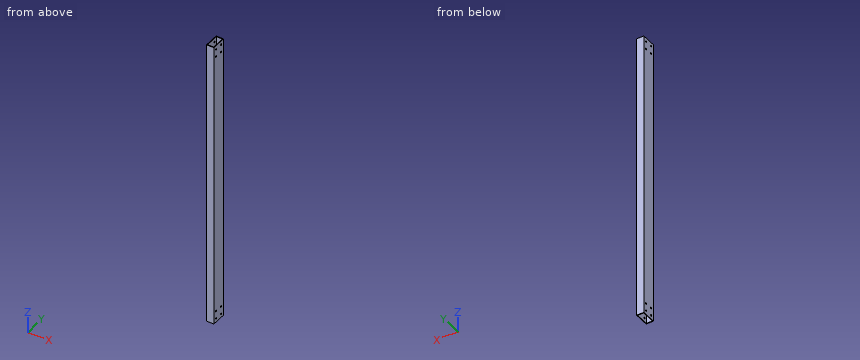
```python
from build123d import *

# Parameters (mm, degrees)
SKETCH1_W                = 38.1
SKETCH1_H                = 76.2
SKETCH1_W_2              = 31.75
SKETCH1_H_2              = 69.85
EXTRUDE_THIN1_DEPTH      = 760
M8_CLEARANCE_HOLE2_D     = 9
M8_CLEARANCE_HOLE2_DEPTH = 3.175
M8_CLEARANCE_HOLE1_D     = 9


with BuildPart() as part:
    # Sketch1 → Extrude-Thin1 (new, symmetric)
    with BuildSketch(Plane.XY):
        Rectangle(SKETCH1_W, SKETCH1_H)
        Rectangle(SKETCH1_W_2, SKETCH1_H_2, mode=Mode.SUBTRACT)
    extrude(amount=EXTRUDE_THIN1_DEPTH, both=True)

    # M8 Clearance Hole2
    with Locations(Plane(origin=(19.05, 0, 0), x_dir=(0, 0, -1), z_dir=(1, 0, 0))):
        with Locations((-740, 20), (-740, -20), (-700, 20), (-700, -20)):
            m8_clearance_hole2 = Hole(M8_CLEARANCE_HOLE2_D / 2, depth=M8_CLEARANCE_HOLE2_DEPTH)

    # M8 Clearance Hole1 (through all)
    with Locations(Plane(origin=(-15.875, 0, 0), x_dir=(0, 0, -1), z_dir=(1, 0, 0))):
        with Locations((-740, 20), (-740, -20), (-700, 20), (-700, -20)):
            m8_clearance_hole1 = Hole(M8_CLEARANCE_HOLE1_D / 2)

    # Mirror1: M8 Clearance Hole2, M8 Clearance Hole1 across plane
    add(m8_clearance_hole2.mirror(Plane.XY), mode=Mode.SUBTRACT)
    add(m8_clearance_hole1.mirror(Plane.XY), mode=Mode.SUBTRACT)


solid = part.part
```
Input: part model. Units: mm. Frame: model coordinates. Give positions to 0.01 mm unless a question says otherwise; leave off trailing zeros. Order: outer loops, then holes, each group sorted by start corner. A loop starts at its lowest first (then second) coordinate and runs counter-clockwise, first axis right, second up.
1. Section A-A on x = 5.5. Return the cut outline in (y, z) (3 decimals).
Derived:
outline: (-38.1, -760) - (-34.925, -760) - (-34.925, 760) - (-38.1, 760) - close; (34.925, -760) - (38.1, -760) - (38.1, 760) - (34.925, 760) - close
2. Section B-B on z = -145. Return the cut outline in (x, y) (3 decimals), and give its area (3 significant figures).
Derived:
outline: (-19.05, -38.1) - (19.05, -38.1) - (19.05, 38.1) - (-19.05, 38.1) - close; hole (-15.875, -34.925) - (15.875, -34.925) - (15.875, 34.925) - (-15.875, 34.925) - close
area: 685 mm2
3. Material intervals for L1, parallel to Y at x = -17, z = -740; L2, parallel to Y at x = -11, z = 315 (3 decimals); L3, parallel to X at y = 10, z = -122 (3 decimals), sorted ascending.
Derived:
L1: y = -38.1 to -24.5, -15.5 to 15.5, 24.5 to 38.1
L2: y = -38.1 to -34.925, 34.925 to 38.1
L3: x = -19.05 to -15.875, 15.875 to 19.05
